Read the model definition and answer for the solid it produces. Units are mm, in the model's axes. Face numbers are marked on the shaded views. A direction names the side the tool comes from. Give positions to 0.01 mm unless a question says otherwise; leave off trailing zeros. Write each loop counter-clockwise with the first axis right and the second up, starting at its lowest first coordinate (ties: lowest second). Pieces come first, ordered by that corner, then holes. Notation, with made-up numbers: (59.25, 40) - (67.25, 40) arc R27 ccw to (67.25, 57) - close; hole circle Ø6 at (-40, 73). An arc over 180 degrees is marked (long way). Answer as CSV lines item,"result".
Autodesk Inventor part; units mm, degrees
ref_plane "YZ Plane" through (0, 0, 0) normal (1, 0, 0) x (0, 1, 0)
ref_plane "XZ Plane" through (0, 0, 0) normal (0, 1, 0) x (-1, 0, 0)
ref_plane "XY Plane" through (0, 0, 0) normal (0, 0, 1) x (1, 0, 0)
sketch "Sketch1" plane through (0, 0, 0) normal (0, 0, 1) x (1, 0, 0)
  arc A0 (-100.8031, -12.7) -> (0, -101.6) centre (0, 0) ccw
  line L0 (0, -101.6) -> (152.4, -101.6)
  line L1 (152.4, -101.6) -> (152.4, -127)
  line L2 (149.225, -104.775) -> (0, -104.775)
  arc A1 (-103.5654, -15.875) -> (0, -104.775) centre (0, 0) ccw
  line L3 (-100.8031, -12.7) -> (-126.2031, -12.7)
  line L4 (-126.2031, -12.7) -> (-126.2031, -15.875)
  line L5 (-126.2031, -15.875) -> (-103.5654, -15.875)
  line L6 (-126.2031, -12.7) -> (-100.8031, -12.7)
  line L7 (-100.8031, -12.7) -> (-100.8031, 0)
  line L8 (-100.8031, 0) -> (-126.2031, 0)
  line L9 (-126.2031, 0) -> (-126.2031, -12.7)
  line L10 (-100.8031, 0) -> (0, 0) construction
  line L11 (149.225, -104.775) -> (149.225, -127)
  line L12 (149.225, -127) -> (152.4, -127)
  dimension "d0" = 25.4
  dimension "d2" = 3.175
  dimension "d3" = 3.175
  dimension "d4" = 12.7
  dimension "d5" = 101.6
  dimension "d6" = 152.4
  dimension "d7" = 3.175
  dimension "d8" = 25.4
extrude "Extrusion1" add sketch "Sketch1" along normal blind 304.8 contours A0 L0 L1 L12 L11 L2 A1 L5 L4 L3
properties part number "Panel_FrontVerticalConveyorShroud_Upper" material "Polycarbonate, Smoke"
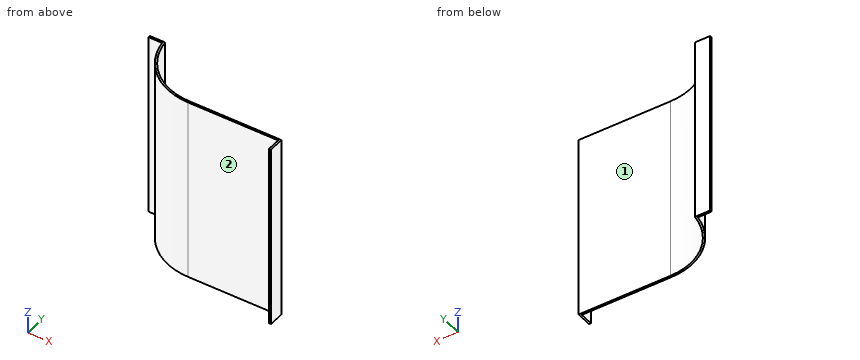
(1) A cutting plane is placed at A-A (z = 20.5). Write down the section's boundary in (x, y) (3 decimals), and give its area (3 significant figures).
Worked out:
outline,"(-126.203, -15.875) - (-103.565, -15.875) arc R104.775 ccw to (0, -104.775) - (149.225, -104.775) - (149.225, -127) - (152.4, -127) - (152.4, -101.6) - (0, -101.6) arc R101.6 cw to (-100.803, -12.7) - (-126.203, -12.7) - close"
area,"1,100 mm^2"
(2) For the marked faces 1 and 2, determine the directions among +Z, -Z, +X, -X, +Y, -Y from which every point of the face is accessible in a straight line to the end or side of a thin tool.
Worked out:
face 1,"+Z, -Z, +X, +Y"
face 2,"+Z, -Z, -X, -Y"
(3) A cutting plane is placed at B-B (x = 6.5). Write down the section's boundary in (y, z) (3 decimals).
Worked out:
outline,"(-104.775, 0) - (-101.6, 0) - (-101.6, 304.8) - (-104.775, 304.8) - close"
(4) Each of these flat-tipped pins is pushed along its axis until it touches: P1, Ø5, axis at y = -33, z = 172, coming from the -X side; P2, Ø6, axis at y = -108, z = 119.5, coming from the -X side (3 decimals); P3, Ø12, axis at y = -27, z = 219, coming from the -X side. Where does it stop, or does it pass through?
Worked out:
P1,"stops at x = -100.24"
P2,"stops at x = 149.225"
P3,"stops at x = -102.65"
(5) Find the intervals of material crossed by L1, parallel to Y at x = 10.5, z = 201 (3 decimals); L2, parallel to X at y = -112.5, z = 124 (3 decimals); L3, parallel to X at y = -36.5, z = 59, in increasing order.
Worked out:
L1,"y = -104.775 to -101.6"
L2,"x = 149.225 to 152.4"
L3,"x = -98.21 to -94.82"
(6) A cutting plane is placed at C-C (y = -29.5). Write down the section's boundary in (x, z), and give its area (3 significant figures).
Worked out:
outline,"(-100.54, 0) - (-97.22, 0) - (-97.22, 304.8) - (-100.54, 304.8) - close"
area,"1,010 mm^2"
